Verification items for the finished model (mm, model axes). A direction names the side the tool comes from. Give positions to 0.01 mm unless a question says otherwise; leave off trailing zeros. Loops run counter-clockwise (first coordinate to the right, second up) from the corner with the lowest first, then second, coordinate; pieces in that order, holes last. Notation, with made-up numbers: M 39.25,61 L 52.25,61 A31 cw 52.25,91 Z; hole C 43,-31.75 d1. An arc over 180 degrees is marked long. Use CSV: the item, a comma, the result in double quotes.
from build123d import *

# Parameters (mm, degrees)
SKETCH_1_W      = 1200
SKETCH_1_H      = 600
EXTRUDE_1_DEPTH = 30
SKETCH_2_W      = 50
SKETCH_2_H      = 50
EXTRUDE_2_DEPTH = 750
SKETCH_3_W      = 50
SKETCH_3_H      = 50
EXTRUDE_3_DEPTH = 750
SKETCH_4_W      = 50
SKETCH_4_H      = 50
EXTRUDE_4_DEPTH = 750
SKETCH_5_W      = 50
SKETCH_5_H      = 50
EXTRUDE_5_DEPTH = 750


with BuildPart() as part:
    # 草图1 → 凸台-拉伸1 (new body)
    with BuildSketch(Plane.XY):
        Rectangle(SKETCH_1_W, SKETCH_1_H)
    extrude(amount=EXTRUDE_1_DEPTH)

    # 草图2 → 凸台-拉伸2 (add)
    with BuildSketch(Plane.XY):
        with Locations((-550, -250)):
            Rectangle(SKETCH_2_W, SKETCH_2_H)
    extrude(amount=EXTRUDE_2_DEPTH)

    # 草图3 → 凸台-拉伸3 (add)
    with BuildSketch(Plane.XY):
        with Locations((550, -250)):
            Rectangle(SKETCH_3_W, SKETCH_3_H)
    extrude(amount=EXTRUDE_3_DEPTH)

    # 草图4 → 凸台-拉伸4 (add)
    with BuildSketch(Plane.XY):
        with Locations((-550, 250)):
            Rectangle(SKETCH_4_W, SKETCH_4_H)
    extrude(amount=EXTRUDE_4_DEPTH)

    # 草图5 → 凸台-拉伸5 (add)
    with BuildSketch(Plane.XY):
        with Locations((550, 250)):
            Rectangle(SKETCH_5_W, SKETCH_5_H)
    extrude(amount=EXTRUDE_5_DEPTH)


solid = part.part
(1) Section check C-C on x = 419. Record the cut outline in (y, z).
Calculated:
outline,"M -300,0 L 300,0 L 300,30 L -300,30 Z"
(2) Mould release check, pull along Y, two halves, no side actions. Record for faces 1 (the flat face through (-550, -225, 385)), 2 (the flat face through (550, 250, 750)), 3 (the flat face through (550, 275, 385)): released by +Y, released by -Y, zero draft, split by the parting line, or undercut.
Calculated:
face 1,"undercut"
face 2,"zero draft"
face 3,"released by +Y"
(3) Depth check by flat-ended pin: pin 1 Ø15 at (y, z) = (-248, 260.5) entering from +X; pin 2 Ø25 at (x, z) = (-554.5, 567.5) entering from -Y; pin 3 Ø25 at (x, z) = (-548.5, 312) entering from +Y. Enter the tip coordinate at first touch or a pass-through.
Calculated:
pin 1,"stops at x = 575"
pin 2,"stops at y = -275"
pin 3,"stops at y = 275"
(4) Scan lines: L1, parallel to X at y = -261.5, z = 56.5; L2, parallel to Z at x = 345.5, y = 130.5. Record each from-to range of solid material in increasing order. Write a range as from..to.
Calculated:
L1,"x = -575..-525, 525..575"
L2,"z = 0..30"
(5) Section check A-A on z = 391. Record the cut outline in (x, y).
Calculated:
outline,"M -575,-275 L -525,-275 L -525,-225 L -575,-225 Z; M -575,225 L -525,225 L -525,275 L -575,275 Z; M 525,-275 L 575,-275 L 575,-225 L 525,-225 Z; M 525,225 L 575,225 L 575,275 L 525,275 Z"
(6) Section check B-B on y = -253. Record the cut outline in (x, z).
Calculated:
outline,"M -600,0 L 600,0 L 600,30 L 575,30 L 575,750 L 525,750 L 525,30 L -525,30 L -525,750 L -575,750 L -575,30 L -600,30 Z"
(7) Tool access check on faces 4 (the flat face through (-550, -275, 385)), 5 (the flat face through (-575, 250, 385)), 6 (the flat face through (525, -250, 385)). Record the directions out of +Z, -Z, +X, -X, +Y, -Y that give a thin tool (end or side, any length) a straight path to the whole face; none if there is none.
Calculated:
face 4,"+Z, +X, -X, -Y"
face 5,"+Z, -X, +Y, -Y"
face 6,"+Z, +Y, -Y"
